Source: three-view drawing plus pictorial views. Frame: mm from the lowest corner of the part. Give positions to 0.01 mm unless a question says otherwise; leave off trailing zeros. Order: outer loops, then holes, each group sorted by start corner. A loop starts at its lowest first (then second) coordinate and runs counter-clockwise, first axis right, second up. Notation, with made-up numbers: M 23.25,84.5 L 65.25,84.5 A30 ccw 65.25,116.5 Z; hole C 46,-12 d10. An arc over 180 degrees is marked long. Use CSV: the item, a comma, the result in double quotes. Start each with the question number.
Item 1: First-contact query: pin 1 (4 mm diameter, centred on y = 127, z = 54, fed in from -X); pin 2 (8 mm diameter, centred on x = 67, z = 145.5, fed in from -Y); pin 3 (6 mm diameter, centred on x = 58, z = 26, fed in from +Y). Flat tips, straight axial feed; report the tip coordinate or a pass-through.
Item 2: Ray query, probe 1 along Y at (x, z) = (71, 35) (1 decimal); probe 2 along X at (y, z) = (71, 27) (1 decimal); probe 3 along Y at (x, z) = (71, 5). Return the intervals inside material, ascending. Write a range as from..to.
Item 3: Pull-direction query (Y, two-part tool) for the marked faces 1, 2 and 3; classes: +Y half, -Y half, draft (parallel to the pull), parting line (faces both ways), or undercut.
Item 4: Section query C-C on z = 79. Return loops of the section in (x, y) (1 decimal), and give its area (3 significant figures).
Item 5: Section query B-B on z = 124. Return loops of the section in (x, y) (1 decimal), and give its area (4 significant figures).
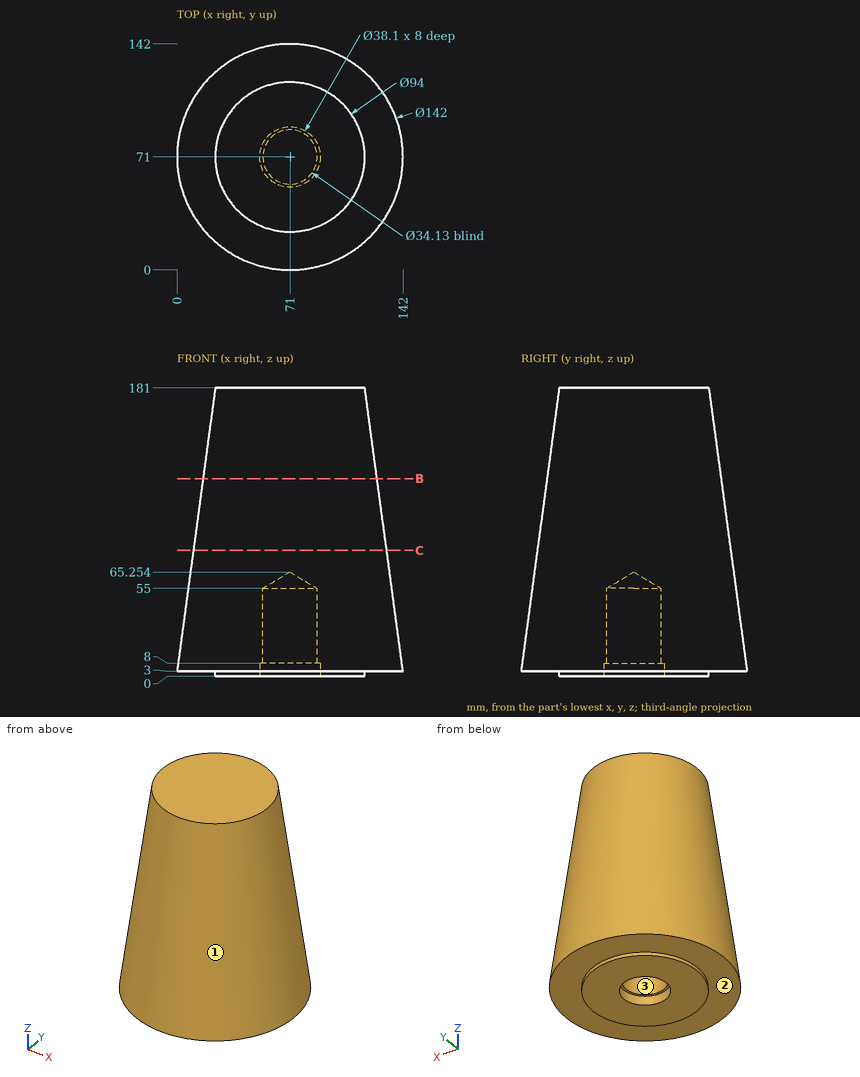
Verdict:
1,pin 1,"x = 36.38"
1,pin 2,"y = 18.77"
1,pin 3,"y = 138.31"
2,probe 1,"4.3..53.9, 88.1..137.7"
2,probe 2,"3.2..53.9, 88.1..138.8"
2,probe 3,"0.27..51.95, 90.05..141.73"
3,face 1,"parting line"
3,face 2,"draft"
3,face 3,"undercut"
4,outline,"C 71,71 d121.5"
4,area,"11,600 mm2"
5,outline,"C 71,71 d109.4"
5,area,"9,395 mm2"
